Could you check a few things on this drawing? It's one solid part, dimensions in mm from its lowest x, y, z. Give positions to 0.01 mm unless a question says otherwise; leave off trailing zeros. Loops run counter-clockwise (first coordinate to the right, second up) from the corner with the lowest first, then second, coordinate; pieces in that order, holes last.
Q1. I need wall thicknesses on probe 1 along Y at (x, z) = (10.16, 3.5); probe 2 along Y at (x, z) = (2.54, 4.75); probe 3 along X at (y, z) = (8.25, 10.5). Which ranges of each line are inside material? Lowest first, please.
Q2. Suppose I cut it at A-A (y = 7.62). List the corners of the cut face in (x, z) for me.
Q3. Suppose I cut it at C-C (z = 3.25). List the corners of the cut face in (x, y) for me, and give its area (3 significant figures).
Q4. Thinking about a two-plate mould opening in X: for the marked faces 1, 2, 3 and 4, which applies, pulls with the +X half, pulls with the -X half, needs draft (parallel to the pull), parting line crosses it, or undercut?
Q5. I'm going to push a flat-ended pin straight in: P1, Ø1.2, axis at x = 10.16, y = 7.62, coming from the -Z side. Where does the tip first touch, or does it pass through?
Q6. Suppose I cut it at B-B (x = 2.54). List the corners of the cut face in (y, z) for me.
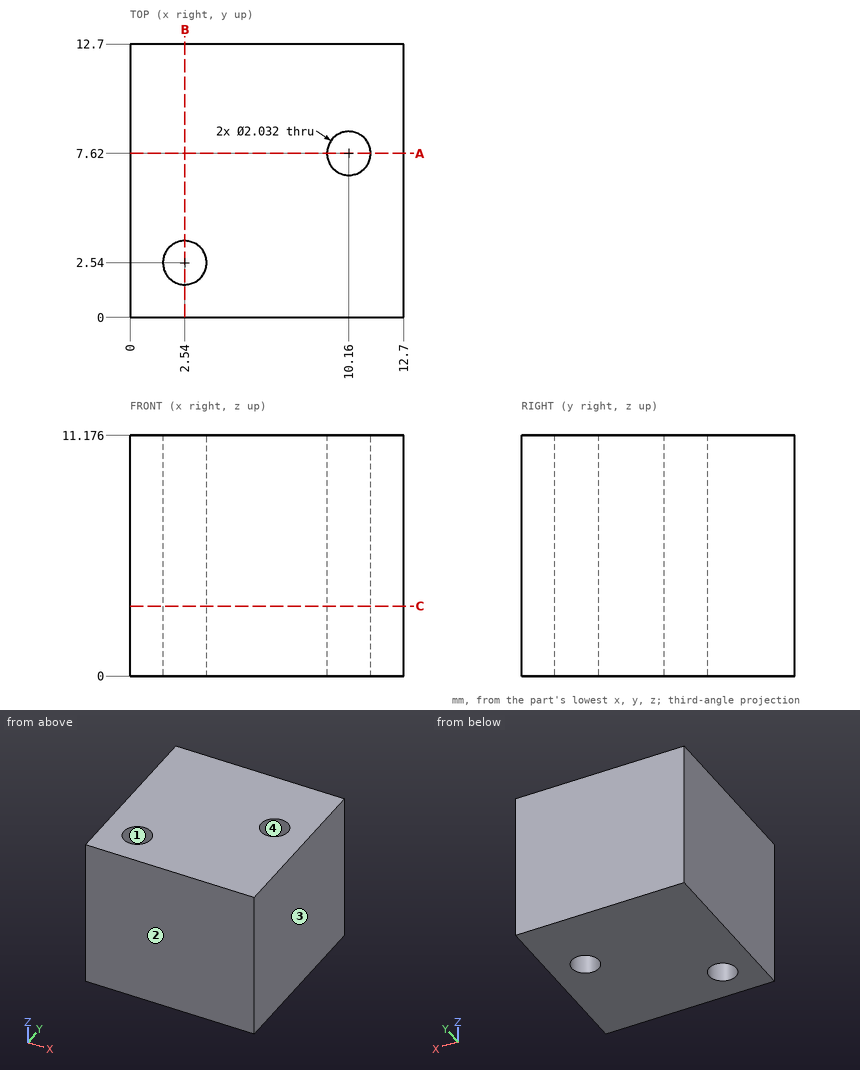
Solutions:
1. probe 1: y = 0 to 6.6, 8.64 to 12.7
1. probe 2: y = 0 to 1.52, 3.56 to 12.7
1. probe 3: x = 0 to 9.36, 10.96 to 12.7
2. outline: (0, 0) - (9.14, 0) - (9.14, 11.18) - (0, 11.18) - close; (11.18, 0) - (12.7, 0) - (12.7, 11.18) - (11.18, 11.18) - close
3. outline: (0, 0) - (12.7, 0) - (12.7, 12.7) - (0, 12.7) - close; hole circle Ø2.03 at (2.54, 2.54); hole circle Ø2.03 at (10.16, 7.62)
3. area: 155 mm2
4. face 1: undercut
4. face 2: needs draft
4. face 3: pulls with the +X half
4. face 4: undercut
5. P1: passes through
6. outline: (0, 0) - (1.52, 0) - (1.52, 11.18) - (0, 11.18) - close; (3.56, 0) - (12.7, 0) - (12.7, 11.18) - (3.56, 11.18) - close
